Verification items for the finished model (mm, model axes). Face numbers are marked on the shaded views. A direction names the side the tool comes from. Coordinates: 2 decimals unless noted, no trailing zeros. Order: outer loops, then holes, each group sorted by start corner. A loop starts at its lowest first (then second) coordinate and runs counter-clockwise, first axis right, second up. Notation, with made-up numbers: M -3.5,37.25 L 19.5,37.25 A19 ccw 19.5,62.25 Z; hole C 7.5,8.5 d11. An arc over 180 degrees is marked long. Return JSON: item names as keys, results as strings. Group by question number.
Q1. Access from +Z, -Z, +X, -X, +Y, -Y to the whole of each face (thin tool, end or side, straight path). Record for the marked faces 1, 2 and 3.
Q2. Section check C-C, the plane z = 1.25. Enter the section's corners in (x, y).
Q3. Thickness scan on probe 1 along X at (y, z) = (-0.5, -0.5); probe 2 along Z at (x, y) = (-2.75, 18.5); probe 3 along Y at (x, z) = (-9, 0.2). Record the ranges inside material, lowest first.
Q4. Go/stop test with flat-tipped pins: pin 1 Ø2.5 at (x, y) = (4, 20) entering from +Z; pin 2 Ø1.4 at (x, z) = (8.5, -4) entering from +Y; pin 3 Ø4 at (x, z) = (-3, 0.5) entering from -Y. Record where each tip stops, or that it passes through.
Q5. Section check D-D, the plane y = 22.5. Enter the section's corners in (x, z), then the cut area to 3 significant figures.
Q6. Section check A-A, the plane z = -0.5. Enter the section's corners in (x, y).
Q7. Section check B-B, the plane x = -1. Enter the section's corners in (y, z), then the cut area to 3 significant figures.
Q8. Mould release check, pull along Y, two halves, no side actions. Record for the marked faces 4, 5 and 6: pulls with the +Y half, pulls with the -Y half, needs draft (parallel to the pull), parting line crosses it, or undercut.
Autodesk Inventor part; units mm, degrees
ref_plane "YZ Plane" through (0, 0, 0) normal (1, 0, 0) x (0, 1, 0)
ref_plane "XZ Plane" through (0, 0, 0) normal (0, 1, 0) x (-1, 0, 0)
ref_plane "XY Plane" through (0, 0, 0) normal (0, 0, 1) x (1, 0, 0)
sketch "Boceto1" plane through (0, 0, 0) normal (0, 0, 1) x (1, 0, 0)
  line L0 (-8, 26.74) -> (8, 26.74)
  line L1 (8, 26.74) -> (8, 0)
  line L2 (8, 0) -> (-8, 0)
  line L3 (-8, 0) -> (-8, 26.74)
  line L4 (6.17, 7.0485) -> (11.67, 7.0485)
  line L5 (11.67, 7.0485) -> (11.67, -3)
  line L6 (11.67, -3) -> (6.17, -3)
  line L7 (6.17, -3) -> (6.17, 7.0485)
  line L8 (-11.67, 7.0485) -> (-6.17, 7.0485)
  line L9 (-6.17, 7.0485) -> (-6.17, -3)
  line L10 (-6.17, -3) -> (-11.67, -3)
  line L11 (-11.67, -3) -> (-11.67, 7.0485)
  circle A0 centre (-9, 10) radius 1
  circle A1 centre (9, 10) radius 1
  circle A2 centre (-9, 10) radius 3.98
  circle A3 centre (9, 10) radius 3.98
  point P0 (0, 0)
  point P1 (0, 0)
  dimension "d0" = 16
  dimension "d1" = 26.74
  dimension "d2" = 5.5
  dimension "d3" = 23.34
  dimension "d6" = 11.67
  dimension "d7" = 29.74
  dimension "d8" = 2
  dimension "d9" = 25.96
  dimension "d10" = 13
extrude "Extrusión1" add sketch "Boceto1" along normal blind 0.74
sketch "Boceto2" plane through (0, 0, 0.74) normal (0, 0, 1) x (1, 0, 0)
  line L0 (-8, 26.74) -> (8, 26.74)
  line L1 (8, 26.74) -> (8, 17.62)
  line L2 (8, 17.62) -> (-8, 17.62)
  line L3 (-8, 17.62) -> (-8, 26.74)
  point P0 (0, 0)
  dimension "d13" = 9.12
extrude "Extrusión2" add sketch "Boceto2" along normal blind 1.82
sketch "Boceto3" plane through (0, 0, 0.74) normal (0, 0, 1) x (1, 0, 0)
  line L0 (9.5, 4.2) -> (10.88, 4.2)
  line L1 (10.88, 4.2) -> (10.88, -1.1)
  line L2 (10.88, -1.1) -> (9.5, -1.1)
  line L3 (9.5, -1.1) -> (9.5, 4.2)
  line L4 (-10.88, 4.2) -> (-9.5, 4.2)
  line L5 (-9.5, 4.2) -> (-9.5, -1.1)
  line L6 (-9.5, -1.1) -> (-10.88, -1.1)
  line L7 (-10.88, -1.1) -> (-10.88, 4.2)
  line L8 (-11.67, 7.0485) -> (-11.67, -3)
  line L9 (6.17, -3) -> (11.67, -3)
  point P0 (0, 0)
  dimension "d16" = 5.3
  dimension "d17" = 1.38
  dimension "d18" = 19
  dimension "d19" = 0.79
  dimension "d20" = 7.2
extrude "Extrusión3" add sketch "Boceto3" along normal blind 2.63
sketch "Boceto4" plane through (0, 0, 0) normal (0, 0, -1) x (-1, 0, 0)
  line L0 (-6.78, -2.6) -> (-11.54, -2.6)
  line L1 (-11.54, -2.6) -> (-11.54, 5.54)
  line L2 (-11.54, 5.54) -> (-6.78, 5.54)
  line L3 (-6.78, 5.54) -> (-6.78, -2.6)
  line L4 (11.54, -2.6) -> (6.78, -2.6)
  line L5 (6.78, -2.6) -> (6.78, 5.54)
  line L6 (6.78, 5.54) -> (11.54, 5.54)
  line L7 (11.54, 5.54) -> (11.54, -2.6)
  line L8 (8, 26.74) -> (-8, 26.74)
  point P0 (0, 0)
  dimension "d23" = 4.76
  dimension "d24" = 23.08
  dimension "d25" = 29.34
  dimension "d26" = 11.54
  dimension "d27" = 8.14
extrude "Extrusión4" add sketch "Boceto4" along normal blind 6.03
shell "Vaciado1" thickness 0.65 removed faces 2 at (8.3667, 0.1133, -6.03) at (-8.3667, 2.8267, -6.03)
properties part number "Encoder" material "Plástico ABS"
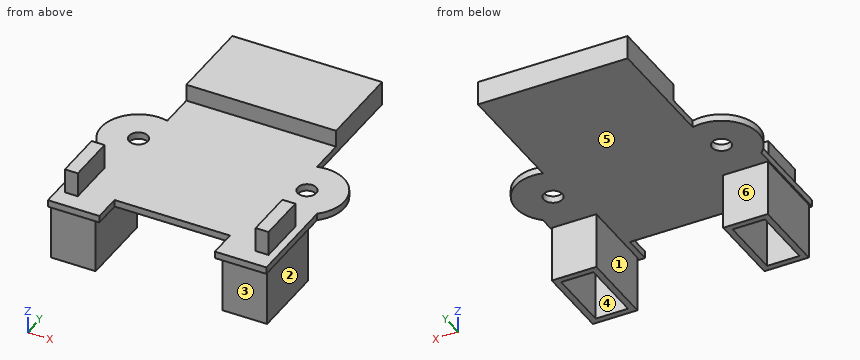
Numbers:
{
 "1": {"face 1": "-Z, +Y, -Y", "face 2": "-Z, +X, +Y, -Y", "face 3": "-Z, +X, -X, -Y"},
 "2": {"outline": "M -10.88,-1.1 L -9.5,-1.1 L -9.5,4.2 L -10.88,4.2 Z; M -8,17.62 L 8,17.62 L 8,26.74 L -8,26.74 Z; M 9.5,-1.1 L 10.88,-1.1 L 10.88,4.2 L 9.5,4.2 Z; hole M -10.23,-0.45 L -10.15,-0.45 L -10.15,3.55 L -10.23,3.55 Z; hole M -7.35,18.27 L 7.35,18.27 L 7.35,26.09 L -7.35,26.09 Z; hole M 10.15,-0.45 L 10.23,-0.45 L 10.23,3.55 L 10.15,3.55 Z"},
 "3": {"probe 1": "x = -11.54 to -10.89, -7.43 to -6.78, 6.78 to 7.43, 10.89 to 11.54", "probe 2": "z = 0 to 0.65, 1.91 to 2.56", "probe 3": "y = -3 to 9, 11 to 13.98"},
 "4": {"pin 1": "stops at z = 2.56", "pin 2": "stops at y = 5.54", "pin 3": "stops at y = 0"},
 "5": {"outline": "M -8,0 L 8,0 L 8,2.56 L -8,2.56 Z; hole M -7.35,0.65 L 7.35,0.65 L 7.35,1.91 L -7.35,1.91 Z", "area": "22.4 mm2"},
 "6": {"outline": "M -11.54,-2.6 L -6.78,-2.6 L -6.78,5.54 L -11.54,5.54 Z; M 6.78,-2.6 L 11.54,-2.6 L 11.54,5.54 L 6.78,5.54 Z; hole M -10.89,-1.95 L -7.43,-1.95 L -7.43,4.89 L -10.89,4.89 Z; hole M 7.43,-1.95 L 10.89,-1.95 L 10.89,4.89 L 7.43,4.89 Z"},
 "7": {"outline": "M 0,0 L 26.74,0 L 26.74,2.56 L 17.62,2.56 L 17.62,0.74 L 0,0.74 Z; hole M 18.27,0.65 L 26.09,0.65 L 26.09,1.91 L 18.27,1.91 Z", "area": "26.5 mm2"},
 "8": {"face 4": "undercut", "face 5": "needs draft", "face 6": "pulls with the +Y half"}
}
